from build123d import *

# Parameters (mm, degrees)
F0_W      = 184.15
F0_H      = 152.4
F1_DEPTH  = 12.7
F3_R      = 3.96875
F4_DEPTH  = 25.4
F5_W      = 25.4
F5_H      = 50.8
F6_DEPTH  = 6.35
F7_W      = 6.35
F7_H      = 50.8
F8_DEPTH  = 44.45
F9_W      = 6.35
F9_H      = 50.8
F10_DEPTH = 44.45


with BuildPart() as f1:
    # F0 (on Top) → F1 (new body)
    with BuildSketch(Plane.XY):
        with Locations((92.075, 76.2)):
            Rectangle(F0_W, F0_H)
    extrude(amount=F1_DEPTH)

    # F3 (on face) → F4 (cut)
    with BuildSketch(Plane(origin=(0, 0, 0), x_dir=(1, 0, 0), z_dir=(0, 0, -1))):
        with Locations((92.075, -82.55)):
            Circle(F3_R)
    extrude(amount=-F4_DEPTH, mode=Mode.SUBTRACT)

    # F5 (on face) → F6 (join)
    with BuildSketch(Plane.XY.offset(12.7)):
        with Locations((12.7, 76.2)):
            Rectangle(F5_W, F5_H)
        with Locations((171.45, 76.2)):
            Rectangle(F5_W, F5_H)
    extrude(amount=F6_DEPTH)

    # F7 (on face) → F8 (join)
    with BuildSketch(Plane.XY.offset(19.05)):
        with Locations((3.175, 76.2)):
            Rectangle(F7_W, F7_H)
    extrude(amount=F8_DEPTH)

    # F9 (on face) → F10 (join)
    with BuildSketch(Plane.XY.offset(19.05)):
        with Locations((180.975, 76.2)):
            Rectangle(F9_W, F9_H)
    extrude(amount=F10_DEPTH)


solid = f1.part
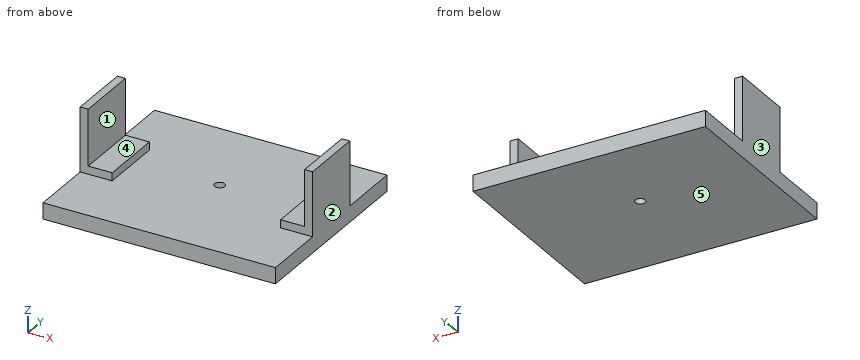
Source: CAD feature listing. Evaluate the final solid. Frame: model axes, mm. Face numbers are marked on the shaded views. A direction names the side the tool comes from. Round coordinates to 2 decimals unless told otherwise and drop trailing zeros. Loops run counter-clockwise (first coordinate to the right, second up) from the corner with the lowest first, then second, coordinate; pieces in that order, holes last.
Q1. Section C-C, the plane x = 73. Return loops of the section in (y, z), plus the area to 3 significant figures.
Q2. Section B-B, the plane z = 16. Return loops of the section in (x, y), plus the area to 3 significant figures.
Q3. Section D-D, the plane y = 117.5. Return loops of the section in (x, z).
Q4. Mould query, pull axis X, two halves, no side actions, for the marked faces 3, 4 and 5. Classes: pulls with the +X half, pulls with the -X half, needs draft (parallel to the pull), parting line crosses it, or undercut.
Q5. First-contact query: P1, Ø1.9, axis at y = 66.5, z = 15.5, coming from the -X side; P2, Ø6, axis at x = 148, y = 35.5, coming from the +Z side; P3, Ø12.5, axis at x = 172.5, z = 39.5, coming from the -Y side; P4, Ø5, axis at x = 158, y = 54.5, coming from the +Z side. Flat tips, straight axial feed; report the tip coordinate or a pass-through.
Q6. Section A-A, the plane y = 82.55. Return loops of the section in (x, z), plus the area to 4 significant figures.
Q7. Access query for the marked faces 1 and 2. Directions: +Z, -Z, +X, -X, +Y, -Y. A direction counts if a zero-diameter tool reaches every point of the face in a straight line with its end or side. Return the directions, or none.
Q8. Ray query, line 1 (X direction, y = 82, z = 5); line 2 (Z direction, x = 42, y = 67.5); line 3 (X direction, y = 64.5, z = 29). Return the intervals inside material, ascending.
Solutions:
1. outline: (0, 0) - (152.4, 0) - (152.4, 12.7) - (0, 12.7) - close
1. area: 1,940 mm2
2. outline: (0, 50.8) - (25.4, 50.8) - (25.4, 101.6) - (0, 101.6) - close; (158.75, 50.8) - (184.15, 50.8) - (184.15, 101.6) - (158.75, 101.6) - close
2. area: 2,580 mm2
3. outline: (0, 0) - (184.15, 0) - (184.15, 12.7) - (0, 12.7) - close
4. face 3: pulls with the -X half
4. face 4: undercut
4. face 5: needs draft
5. P1: stops at x = 0
5. P2: stops at z = 12.7
5. P3: stops at y = 50.8
5. P4: stops at z = 19.05
6. outline: (0, 0) - (88.11, 0) - (88.11, 12.7) - (25.4, 12.7) - (25.4, 19.05) - (6.35, 19.05) - (6.35, 63.5) - (0, 63.5) - close; (96.04, 0) - (184.15, 0) - (184.15, 63.5) - (177.8, 63.5) - (177.8, 19.05) - (158.75, 19.05) - (158.75, 12.7) - (96.04, 12.7) - close
6. area: 3,125 mm2
7. face 1: +Z, +Y, -Y
7. face 2: +Z, -Z, +X, +Y, -Y
8. line 1: x = 0 to 88.14, 96.01 to 184.15
8. line 2: z = 0 to 12.7
8. line 3: x = 0 to 6.35, 177.8 to 184.15
